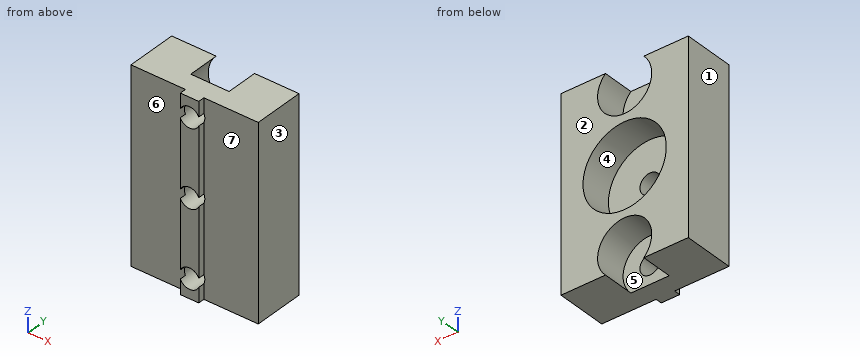
from build123d import *

# Parameters (mm, degrees)
MAIN_DEPTH        = 15
SKETCH5_R         = 1.6
FIXHOLE_DEPTH     = 10
SKETCH3_R         = 6.55
SKETCH3_R_2       = 4.25
BEARINGHOLE_DEPTH = 5


with BuildPart() as part:
    # Sketch1 → Main (new body, symmetric)
    with BuildSketch(Plane.XY):
        Polygon((-10, 9), (10, 9), (10, 1), (1.45, 1), (1.45, 0), (-1.45, 0), (-1.45, 1), (-10, 1), align=None)
    extrude(amount=MAIN_DEPTH, both=True)

    # Sketch5 → FixHole (cut, through all)
    with BuildSketch(Plane(origin=(0, 0, 0), x_dir=(-1, 0, 0), z_dir=(0, -1, 0))):
        with Locations((0, 12)):
            Circle(SKETCH5_R)
        with Locations((0, -12)):
            Circle(SKETCH5_R)
        Circle(SKETCH5_R)
    extrude(amount=-FIXHOLE_DEPTH, mode=Mode.SUBTRACT)

    # Sketch3 → BearingHole (cut)
    with BuildSketch(Plane(origin=(0, 9, 0), x_dir=(1, 0, 0), z_dir=(0, 1, 0))):
        Circle(SKETCH3_R)
        with Locations((0, 12)):
            Circle(SKETCH3_R_2)
        with Locations((0, -12)):
            Circle(SKETCH3_R_2)
    extrude(amount=-BEARINGHOLE_DEPTH, mode=Mode.SUBTRACT)


solid = part.part
Here's how the part is built. I have some questions about the finished solid (model axes, mm). Face numbers are marked on the shaded views. A direction names the side the tool comes from. Round coordinates to 2 decimals unless told otherwise and drop trailing zeros. Write each loop counter-clockwise with the first axis right and the second up, starting at its lowest first coordinate (ties: lowest second). Pieces come first, ordered by that corner, then holes.
1. I need wall thicknesses on L1, parallel to Z at x = 0, y = 0.8; L2, parallel to X at y = 2.3, z = 0; L3, parallel to Z at x = 1, y = 1. Which ranges of each line are inside material? Lowest first, please.
2. If we mould it in two halves opening along X, with no side actions, what happens to the marked faces 1, 2, 3 and 4? For each: released by +X, released by -X, zero draft, split by the parting line, or undercut.
3. Will these pins go through, and if not, where does the flat tip stop? pin 1 Ø8 at (x, z) = (7, 2) entering from -Y; pin 2 Ø0.5 at (y, z) = (0.5, 14.5) entering from -X; pin 3 Ø5 at (x, z) = (0, 0) entering from +Y.
4. Suppose I cut it at C-C (y = 1.5). List the corners of the cut face in (x, z) for me, and give its area (3 significant figures).
5. Suppose I cut it at D-D (y = 5). List the corners of the cut face in (x, z) for me, and give its area (3 significant figures).
6. Suppose I cut it at A-A (x = 0). List the corners of the cut face in (y, z) for me.
7. For the marked faces 5, 6 and 7, which set-ups out of +Z, -Z, +X, -X, +Y, -Y let a thin tool reach every point of the face, with its end or its side?
8. Suppose I cut it at B-B (z = 0). List the corners of the cut face in (x, y) for me.
Answer sheet:
1. L1: z = -15 to -13.6, -10.4 to -1.6, 1.6 to 10.4, 13.6 to 15
1. L2: x = -10 to -1.6, 1.6 to 10
1. L3: z = -15 to -13.25, -10.75 to -1.25, 1.25 to 10.75, 13.25 to 15
2. face 1: released by -X
2. face 2: zero draft
2. face 3: released by +X
2. face 4: undercut
3. pin 1: stops at y = 1
3. pin 2: stops at x = -1.45
3. pin 3: stops at y = 4
4. outline: (-10, -15) - (10, -15) - (10, 15) - (-10, 15) - close; hole circle Ø3.2 at (0, -12); hole circle Ø3.2 at (0, 0); hole circle Ø3.2 at (0, 12)
4. area: 576 mm2
5. outline: (-10, -15) - (-3.01, -15) arc R4.25 cw (long way) to (3.01, -15) - (10, -15) - (10, 15) - (3.01, 15) arc R4.25 cw (long way) to (-3.01, 15) - (-10, 15) - close; hole circle Ø13.1 at (0, 0)
5. area: 362 mm2
6. outline: (0, -15) - (4, -15) - (4, -13.6) - (0, -13.6) - close; (0, -10.4) - (4, -10.4) - (4, -7.75) - (9, -7.75) - (9, -6.55) - (4, -6.55) - (4, -1.6) - (0, -1.6) - close; (0, 1.6) - (4, 1.6) - (4, 6.55) - (9, 6.55) - (9, 7.75) - (4, 7.75) - (4, 10.4) - (0, 10.4) - close; (0, 13.6) - (4, 13.6) - (4, 15) - (0, 15) - close
7. face 5: +Y
7. face 6: +Z, -Z, -X, -Y
7. face 7: +Z, -Z, +X, -Y
8. outline: (-10, 1) - (-1.6, 1) - (-1.6, 4) - (-6.55, 4) - (-6.55, 9) - (-10, 9) - close; (1.6, 1) - (10, 1) - (10, 9) - (6.55, 9) - (6.55, 4) - (1.6, 4) - close
